The listing builds one solid part. Answer for the finished solid, in the listing's coordinates (mm). Round coordinates to 2 decimals unless told otherwise and drop trailing zeros. Loops run counter-clockwise (first coordinate to the right, second up) from the corner with the lowest first, then second, coordinate; pieces in that order, holes last. Notation, with made-up numbers: (-2, -1) - (7, -1) arc R21 cw to (7, 7) - close; hole circle Ø5 at (40.25, 68.5). An arc over 180 degrees is marked (long way). One line per item, written item: value.
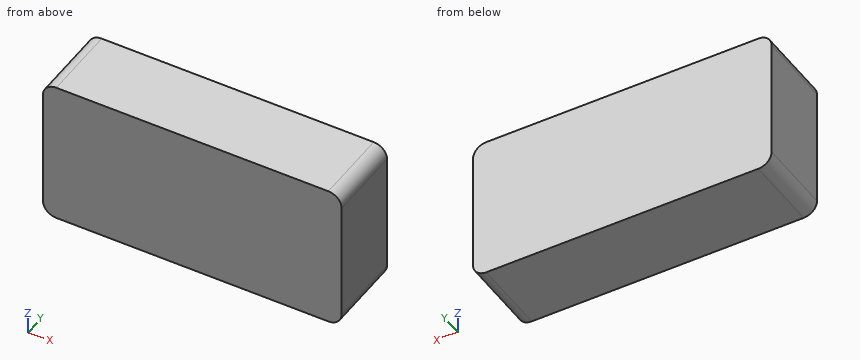
```python
from build123d import *

# Parameters (mm, degrees)
F1_DEPTH = 11.811
F3_DEPTH = 1.4224
F5_DEPTH = 1.4224


with BuildPart() as f1:
    # F0 (on Front) → F1 (new body)
    with BuildSketch(Plane.XZ):
        with BuildLine():
            Line((54.61, 0), (2.54, 0))
            ThreePointArc((2.54, 0), (0.743949, -0.743949), (0, -2.54))
            Line((0, -2.54), (0, -25.4))
            ThreePointArc((0, -25.4), (0.743949, -27.196051), (2.54, -27.94))
            Line((2.54, -27.94), (54.61, -27.94))
            ThreePointArc((54.61, -27.94), (56.406051, -27.196051), (57.15, -25.4))
            Line((57.15, -25.4), (57.15, -2.54))
            ThreePointArc((57.15, -2.54), (56.406051, -0.743949), (54.61, 0))
        make_face()
        with BuildLine():
            ThreePointArc((5.08, -4.2672), (5.451974, -3.369174), (6.35, -2.9972))
            Line((6.35, -2.9972), (50.8, -2.9972))
            ThreePointArc((50.8, -2.9972), (51.698026, -3.369174), (52.07, -4.2672))
            Line((52.07, -4.2672), (52.07, -23.749))
            ThreePointArc((52.07, -23.749), (51.698026, -24.647026), (50.8, -25.019))
            Line((50.8, -25.019), (6.35, -25.019))
            ThreePointArc((6.35, -25.019), (5.451974, -24.647026), (5.08, -23.749))
            Line((5.08, -23.749), (5.08, -4.2672))
        make_face(mode=Mode.SUBTRACT)
    extrude(amount=F1_DEPTH)

    # F2 (on face) → F3 (join)
    with BuildSketch(Plane(origin=(0, 0, 0), x_dir=(-1, 0, 0), z_dir=(0, 1, 0))):
        with BuildLine():
            ThreePointArc((0, -2.54), (-0.743949, -0.743949), (-2.54, 0))
            Line((-2.54, 0), (-54.61, 0))
            ThreePointArc((-54.61, 0), (-56.406051, -0.743949), (-57.15, -2.54))
            Line((-57.15, -2.54), (-57.15, -25.4))
            ThreePointArc((-57.15, -25.4), (-56.406051, -27.196051), (-54.61, -27.94))
            Line((-54.61, -27.94), (-2.54, -27.94))
            ThreePointArc((-2.54, -27.94), (-0.743949, -27.196051), (0, -25.4))
            Line((0, -25.4), (0, -2.54))
        make_face()
    extrude(amount=F3_DEPTH)

    # F4 (on face) → F5 (join)
    with BuildSketch(Plane.XZ.offset(11.811)):
        with BuildLine():
            Line((54.61, 0), (2.54, 0))
            ThreePointArc((2.54, 0), (0.743949, -0.743949), (0, -2.54))
            Line((0, -2.54), (0, -25.4))
            ThreePointArc((0, -25.4), (0.743949, -27.196051), (2.54, -27.94))
            Line((2.54, -27.94), (54.61, -27.94))
            ThreePointArc((54.61, -27.94), (56.406051, -27.196051), (57.15, -25.4))
            Line((57.15, -25.4), (57.15, -2.54))
            ThreePointArc((57.15, -2.54), (56.406051, -0.743949), (54.61, 0))
        make_face()
    extrude(amount=F5_DEPTH)


solid = f1.part
```
1) A cutting plane is placed at B-B on x = 40. Give the vertices of the cut face in (y, z), and give its area (3 significant figures).
Final values:
outline: (-13.23, -27.94) - (1.42, -27.94) - (1.42, 0) - (-13.23, 0) - close; hole (-11.81, -25.02) - (0, -25.02) - (0, -3) - (-11.81, -3) - close
area: 149 mm2
2) A cutting plane is placed at A-A on y = -10. Give the vertices of the cut face in (x, z), and give its area (3 significant figures).
Final values:
outline: (0, -25.4) arc R2.54 ccw to (2.54, -27.94) - (54.61, -27.94) arc R2.54 ccw to (57.15, -25.4) - (57.15, -2.54) arc R2.54 ccw to (54.61, 0) - (2.54, 0) arc R2.54 ccw to (0, -2.54) - close; hole (5.08, -23.75) arc R1.27 ccw to (6.35, -25.02) - (50.8, -25.02) arc R1.27 ccw to (52.07, -23.75) - (52.07, -4.27) arc R1.27 ccw to (50.8, -3) - (6.35, -3) arc R1.27 ccw to (5.08, -4.27) - close
area: 558 mm2
3) A cutting plane is placed at C-C on z = -11.75. Give the vertices of the cut face in (x, y), and give its area (3 significant figures).
Final values:
outline: (0, -13.23) - (57.15, -13.23) - (57.15, 1.42) - (0, 1.42) - close; hole (5.08, -11.81) - (52.07, -11.81) - (52.07, 0) - (5.08, 0) - close
area: 283 mm2
4) Consider L1, parallel to X at y = -8.25, z = -16; L2, parallel to Y at x = 5.5, z = -13; L3, parallel to Z at x = 45, y = -10.25. Determine where each line is inside the solid, lowest interval first.
Final values:
L1: 0 to 5.08, 52.07 to 57.15
L2: -13.23 to -11.81, 0 to 1.42
L3: -27.94 to -25.02, -3 to 0
